Work out the finished part from the listing and answer in its coordinate system (mm). Face numbers are marked on the shaded views. A direction names the side the tool comes from. Give positions to 0.01 mm unless a question says otherwise; leave off trailing zeros. Loops run counter-clockwise (first coordinate to the right, second up) from the corner with the lowest first, then second, coordinate; pieces in that order, holes last. Notation, with made-up numbers: (51, 63.25) -> (108, 63.25) arc R25 cw to (108, 85.25) -> close; hole circle Ø7 at (51.5, 28). An arc over 180 degrees is marked (long way). Answer as CSV lines item,"result". Start each with the question number.
1. Find section D-D, the plane x = -17.5. Give the vertices of the cut face in (y, z).
2. A tool of negligible diameter and unlimited length cuts with its end or side. For the marked faces 4, 5 and 6, from which of +Z, -Z, +X, -X, +Y, -Y can it reach the whole face along a straight path? Write none if from no direction.
3. Find section A-A, the plane y = 2.5. Give the vertices of the cut face in (x, z).
4. Determine the mould class of the marked faces 1, 2 and 3 for opening direction Y: +Y half, -Y half, draft (parallel to the pull), parting line (faces both ways), or undercut.
5. Flat-ended cylindrical pins translate along their axes: pin 1 Ø6.5 at (y, z) = (-15, 11) entering from -X; pin 2 Ø19 at (x, y) = (-6, -9) entering from +Z; pin 3 Ø3.5 at (x, y) = (-7, -14.5) entering from +Z; pin 4 Ø8.5 at (x, z) = (-10.5, 7) entering from +Y. Find the tip coordinate at first contact, or state that the pin passes through.
6. Find section C-C, the plane x = 6. Give the vertices of the cut face in (y, z).
7. Find section B-B, the plane z = 1.5. Give the vertices of the cut face in (x, y), and give its area (3 significant figures).
8. Find the intervals of material crossed by line 1 along Y through (x, z) = (-6.5, 5); line 2 along Z through (x, y) = (-18.5, 1); line 3 along Y through (x, z) = (6, 0.45), in increasing order.
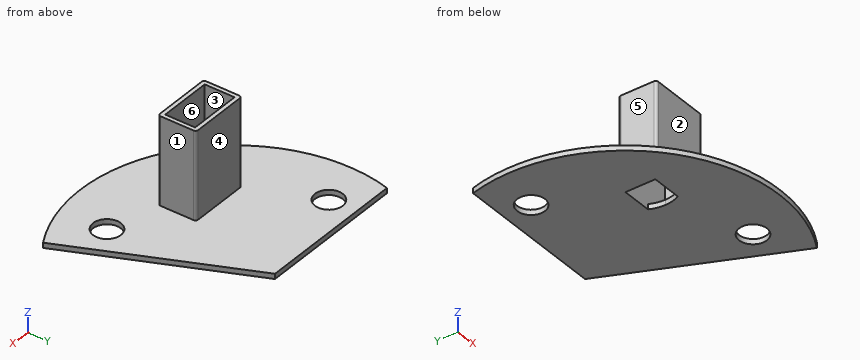
from build123d import *

# Parameters (mm, degrees)
F0_R     = 2.7
F1_DEPTH = 1
F2_DEPTH = 18


# Not quite as in the source:
# - a feature names something its author has since deleted; it is built from what else it names


with BuildPart() as f1:
    # F0 (on Top) → F1 (new body)
    with BuildSketch(Plane.XY):
        with BuildLine():
            Line((0, 7.8000635883), (-28.9682413691, 7.8000635883))
            ThreePointArc((-28.9682413691, 7.8000635883), (-18.3237536434, -23.7537376515), (14.8986014601, -26.039041352))
            Line((14.8986014601, -26.039041352), (0, 7.8000635883))
        make_face()
        with BuildLine():
            ThreePointArc((-9.6558443136, -17.9), (-21.5, -14.2), (-9.6558443136, -10.5))
            Line((-9.6558443136, -10.5), (-4.5, -10.5))
            ThreePointArc((-4.5, -10.5), (-4.1464466094, -10.6464466094), (-4, -11))
            Line((-4, -11), (-4, -17.4))
            ThreePointArc((-4, -17.4), (-4.1464466094, -17.7535533906), (-4.5, -17.9))
            Line((-4.5, -17.9), (-9.6558443136, -17.9))
        make_face(mode=Mode.SUBTRACT)
        with Locations((6, -20.3)):
            Circle(F0_R, mode=Mode.SUBTRACT)
        with Locations((-21, 2.5)):
            Circle(F0_R, mode=Mode.SUBTRACT)
        with BuildLine():
            Line((-15.3, -10.5), (-9.6558443136, -10.5))
            ThreePointArc((-9.6558443136, -10.5), (-21.5, -14.2), (-9.6558443136, -17.9))
            Line((-9.6558443136, -17.9), (-15.3, -17.9))
            ThreePointArc((-15.3, -17.9), (-15.6535533906, -17.7535533906), (-15.8, -17.4))
            Line((-15.8, -17.4), (-15.8, -11))
            ThreePointArc((-15.8, -11), (-15.6535533906, -10.6464466094), (-15.3, -10.5))
        make_face()
        with BuildLine():
            Line((-15, -11.3), (-9.1827841711, -11.3))
            ThreePointArc((-9.1827841711, -11.3), (-9.4049974508, -10.8915341207), (-9.6558443136, -10.5))
            Line((-9.6558443136, -10.5), (-15.3, -10.5))
            ThreePointArc((-15.3, -10.5), (-15.6535533906, -10.6464466094), (-15.8, -11))
            Line((-15.8, -11), (-15.8, -17.4))
            ThreePointArc((-15.8, -17.4), (-15.6535533906, -17.7535533906), (-15.3, -17.9))
            Line((-15.3, -17.9), (-9.6558443136, -17.9))
            ThreePointArc((-9.6558443136, -17.9), (-9.4049974508, -17.5084658793), (-9.1827841711, -17.1))
            Line((-9.1827841711, -17.1), (-15, -17.1))
            Line((-15, -17.1), (-15, -11.3))
        make_face()
        with BuildLine():
            ThreePointArc((-9.6558443136, -10.5), (-9.4049974508, -10.8915341207), (-9.1827841711, -11.3))
            Line((-9.1827841711, -11.3), (-4.8, -11.3))
            Line((-4.8, -11.3), (-4.8, -17.1))
            Line((-4.8, -17.1), (-9.1827841711, -17.1))
            ThreePointArc((-9.1827841711, -17.1), (-9.4049974508, -17.5084658793), (-9.6558443136, -17.9))
            Line((-9.6558443136, -17.9), (-4.5, -17.9))
            ThreePointArc((-4.5, -17.9), (-4.1464466094, -17.7535533906), (-4, -17.4))
            Line((-4, -17.4), (-4, -11))
            ThreePointArc((-4, -11), (-4.1464466094, -10.6464466094), (-4.5, -10.5))
            Line((-4.5, -10.5), (-9.6558443136, -10.5))
        make_face()
        with BuildLine():
            ThreePointArc((-9.1827841711, -11.3), (-8.6729982263, -12.7103528753), (-8.5, -14.2))
            ThreePointArc((-8.5, -14.2), (-8.6729982263, -15.6896471247), (-9.1827841711, -17.1))
            Line((-9.1827841711, -17.1), (-4.8, -17.1))
            Line((-4.8, -17.1), (-4.8, -11.3))
            Line((-4.8, -11.3), (-9.1827841711, -11.3))
        make_face()
    extrude(amount=F1_DEPTH)

    # F0 (on Top) → F2 (join)
    with BuildSketch(Plane.XY):
        with BuildLine():
            Line((-15, -11.3), (-9.1827841711, -11.3))
            ThreePointArc((-9.1827841711, -11.3), (-9.4049974508, -10.8915341207), (-9.6558443136, -10.5))
            Line((-9.6558443136, -10.5), (-15.3, -10.5))
            ThreePointArc((-15.3, -10.5), (-15.6535533906, -10.6464466094), (-15.8, -11))
            Line((-15.8, -11), (-15.8, -17.4))
            ThreePointArc((-15.8, -17.4), (-15.6535533906, -17.7535533906), (-15.3, -17.9))
            Line((-15.3, -17.9), (-9.6558443136, -17.9))
            ThreePointArc((-9.6558443136, -17.9), (-9.4049974508, -17.5084658793), (-9.1827841711, -17.1))
            Line((-9.1827841711, -17.1), (-15, -17.1))
            Line((-15, -17.1), (-15, -11.3))
        make_face()
        with BuildLine():
            ThreePointArc((-9.6558443136, -10.5), (-9.4049974508, -10.8915341207), (-9.1827841711, -11.3))
            Line((-9.1827841711, -11.3), (-4.8, -11.3))
            Line((-4.8, -11.3), (-4.8, -17.1))
            Line((-4.8, -17.1), (-9.1827841711, -17.1))
            ThreePointArc((-9.1827841711, -17.1), (-9.4049974508, -17.5084658793), (-9.6558443136, -17.9))
            Line((-9.6558443136, -17.9), (-4.5, -17.9))
            ThreePointArc((-4.5, -17.9), (-4.1464466094, -17.7535533906), (-4, -17.4))
            Line((-4, -17.4), (-4, -11))
            ThreePointArc((-4, -11), (-4.1464466094, -10.6464466094), (-4.5, -10.5))
            Line((-4.5, -10.5), (-9.6558443136, -10.5))
        make_face()
    extrude(amount=F2_DEPTH)


solid = f1.part
Resolved:
1,outline,"(-24.37, 0) -> (7.8, 0) -> (7.8, 1) -> (-24.37, 1) -> close"
2,face 4,"+Z, +X, -X, +Y"
2,face 5,"+Z, -X, +Y, -Y"
2,face 6,"+Z"
3,outline,"(-29.9, 0) -> (-23.7, 0) -> (-23.7, 1) -> (-29.9, 1) -> close; (-18.3, 0) -> (2.33, 0) -> (2.33, 1) -> (-18.3, 1) -> close"
4,face 1,"draft"
4,face 2,"-Y half"
4,face 3,"undercut"
5,pin 1,"stops at x = -15.8"
5,pin 2,"stops at z = 18"
5,pin 3,"stops at z = 1"
5,pin 4,"stops at y = -10.5"
6,outline,"(-29.39, 0) -> (-23, 0) -> (-23, 1) -> (-29.39, 1) -> close; (-17.6, 0) -> (-5.83, 0) -> (-5.83, 1) -> (-17.6, 1) -> close"
7,outline,"(-15.8, -17.4) arc R0.5 ccw to (-15.3, -17.9) -> (-4.5, -17.9) arc R0.5 ccw to (-4, -17.4) -> (-4, -11) arc R0.5 ccw to (-4.5, -10.5) -> (-15.3, -10.5) arc R0.5 ccw to (-15.8, -11) -> close; hole (-15, -17.1) -> (-4.8, -17.1) -> (-4.8, -11.3) -> (-15, -11.3) -> close"
7,area,"27.9 mm^2"
8,line 1,"y = -17.9 to -17.1, -11.3 to -10.5"
8,line 2,"z = 0 to 1"
8,line 3,"y = -29.39 to -23, -17.6 to -5.83"
